Verification items for the finished model (mm, model axes). A direction names the side the tool comes from. Coordinates: 2 decimals unless noted, no trailing zeros. Write each loop counter-clockwise with the first axis right and the second up, starting at its lowest first coordinate (ties: lowest second). Pieces come first, ordered by that corner, then holes. Notation, with made-up numbers: (16.25, -27.75) -> (39.25, -27.75) arc R23 ccw to (39.25, -15.75) -> close; hole circle Ø9 at (19, -2). An arc over 180 degrees is marked (long way). Answer in a Markdown table with one row per item.
```python
from build123d import *


with BuildPart() as f3:
    # F0 (on Top) → F3 section 0
    with BuildSketch(Plane.XY, mode=Mode.PRIVATE) as f3_s0:
        Polygon((28.473403, 25.65019), (0, 0), (-37.869632, 25.65019), (-28.631995, 3.395881), (-40.844899, -14.635104), (-16.992594, -41.112736), (0, -46.57134), (19.235764, -41.112736), (35.906301, -10.448431), (23.434689, 3.395881), align=None)
    loft([Vertex(0, 0, 100), f3_s0.sketch])


solid = f3.part
```
1. Thickness scan on line 1 (X direction, y = 7, z = 67.5); line 2 (Z direction, x = 24, y = -17); line 3 (Z direction, x = -3, y = -6). Record the ranges inside material, lowest first. Write a range as from..to.
Geometry says:
| item | result |
|---|---|
| line 1 | -11.75..-10.33, 7.77..8.95 |
| line 2 | 0..20.07 |
| line 3 | 0..84.44 |
2. Depth check by flat-ended pin: P1, Ø10, axis at x = 3.5, z = 17.5, coming from the -Y side; P2, Ø12, axis at y = -22.5, z = 77, coming from the +X side; P3, Ø8, axis at y = -30.5, z = 11.5, coming from the -X side; P4, Ø4, axis at x = -16.5, z = 64.5, coming from the +Y side. Enter the tip coordinate at first touch or a pass-through.
Geometry says:
| item | result |
|---|---|
| P1 | y = -40.15 |
| P2 | through |
| P3 | x = -24.54 |
| P4 | y = -5.06 |
3. Section check C-C, the plane x = -20.5. Record the boundary of the cut face in (y, z).
Geometry says:
| item | result |
|---|---|
| outline | (-37.22, 0) -> (13.89, 0) -> (13.89, 45.87) -> (2.43, 28.4) -> (-7.35, 49.81) -> close |
4. Tool access check on faces 1 (the flat face through (19.957, -1.934, 31.248)), 2 (the flat face through (-14.462, 9.796, 38.189)), 3 (the flat face through (-24.353, -4.557, 31.248)). Record the directions out of +Z, -Z, +X, -X, +Y, -Y that give a thin tool (end or side, any length) a straight path to the whole face; none if there is none.
Geometry says:
| item | result |
|---|---|
| face 1 | +Z, +X |
| face 2 | +Z, -Z, +Y |
| face 3 | +Z, -X |
5. Section check A-A, the plane y = 18.5. Record the boundary of the cut face in (x, z), plus the area to 3 significant figures.
Geometry says:
| item | result |
|---|---|
| outline | (-34.9, 0) -> (-27.31, 0) -> (-27.31, 27.88) -> close; (20.54, 0) -> (26.85, 0) -> (20.54, 27.88) -> close |
| area | 194 mm^2 |
6. Section check B-B, the plane z = 89. Record the boundary of the cut face in (x, y).
Geometry says:
| item | result |
|---|---|
| outline | (-4.49, -1.61) -> (-1.87, -4.52) -> (0, -5.12) -> (2.12, -4.52) -> (3.95, -1.15) -> (2.58, 0.37) -> (3.13, 2.82) -> (0, 0) -> (-4.17, 2.82) -> (-3.15, 0.37) -> close |
7. Section check D-D, the plane y = -17. Record the boundary of the cut face in (x, z).
Geometry says:
| item | result |
|---|---|
| outline | (-38.71, 0) -> (32.34, 0) -> (7.95, 58.65) -> (0, 63.5) -> (-7.03, 58.65) -> close |
